Autodesk Inventor part; units mm, degrees
ref_plane "YZ Plane" through (0, 0, 0) normal (1, 0, 0) x (0, 1, 0)
ref_plane "XZ Plane" through (0, 0, 0) normal (0, 1, 0) x (-1, 0, 0)
ref_plane "XY Plane" through (0, 0, 0) normal (0, 0, 1) x (1, 0, 0)
sketch "Sketch1" plane through (0, 0, 0) normal (1, 0, 0) x (0, 1, 0)
  line L0 (6.2348, 11.9337) -> (6.2348, 11.9337)
  line L1 (2.2348, 7.9337) -> (2.2348, -14.0663)
  line L2 (6.2348, -18.0663) -> (6.2348, -18.0663)
  line L3 (10.2348, -14.0663) -> (10.2348, 7.9337)
  circle A0 centre (6.2348, 6.9337) radius 1.25
  circle A1 centre (6.2348, -3.0663) radius 1.25
  circle A2 centre (6.2348, -13.0663) radius 2.25
  arc A3 (6.2348, -18.0663) -> (10.2348, -14.0663) centre (6.2348, -14.0663) ccw
  arc A4 (2.2348, -14.0663) -> (6.2348, -18.0663) centre (6.2348, -14.0663) ccw
  arc A5 (6.2348, 11.9337) -> (2.2348, 7.9337) centre (6.2348, 7.9337) ccw
  arc A6 (10.2348, 7.9337) -> (6.2348, 11.9337) centre (6.2348, 7.9337) ccw
  point P0 (0, 0)
  point P1 (10.2348, 11.9337)
  point P2 (2.2348, 11.9337)
  point P3 (10.2348, -18.0663)
  dimension "d0" = 30
  dimension "d1" = 8
  dimension "d2" = 10
  dimension "d3" = 20
  dimension "d4" = 5
  dimension "d5" = 4.5
  dimension "d6" = 2.5
  dimension "d7" = 2.5
  dimension "d8" = 4
extrude "Extrusion1" add sketch "Sketch1" along normal blind 2
sketch "Sketch2" plane through (2, 0, 0) normal (1, 0, 0) x (0, 0, -1)
  circle A0 centre (-1.9337, 6.2348) radius 2
  circle A1 centre (3.0663, 6.2348) radius 1.25
  point P0 (0, 0)
  dimension "d11" = 4
  dimension "d12" = 5
extrude "Extrusion2" add sketch "Sketch2" along normal blind 10 contours A0
fillet "Fillet1" radius 1 1 edges at (2, 6.2348, 3.9337)
sketch "Sketch4" plane through (2, 0, 0) normal (1, 0, 0) x (0, 0, -1)
  circle A0 centre (13.0663, 6.2348) radius 2.25
  circle A1 centre (13.0663, 6.2348) radius 2.4
  point P0 (0, 0)
  dimension "d25" = 4.8
extrude "Extrusion4" add sketch "Sketch4" along normal blind 9 and the other way blind 2 contours A0
fillet "Fillet2" radius 1 1 edges at (11, 6.2348, -10.8163)
properties part number "cube_Holder"
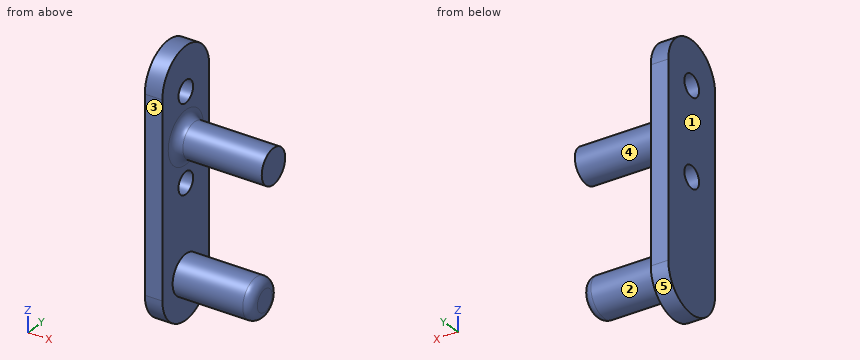
Geometry check sheet. Reference: the model listing, model coordinates, mm. Face numbers are marked on the shaded views. A direction names the side the tool comes from. Round coordinates to 2 decimals unless told otherwise and drop trailing zeros. Loops run counter-clockwise (first coordinate to the right, second up) from the corner with the lowest first, then second, coordinate; pieces in that order, holes last. Notation, with made-up numbers: M -20.5,-10 L 30.5,-10 A30 cw 30.5,13 Z; hole C 7,-29 d1. An arc over 180 degrees is marked long. Return JSON: item names as keys, results as strings. Group by question number.
(1) Section check C-C, the plane y = 5.5. Give the number of separate pieces and of enclosed holes in the cut face, and give its area (3 significant figures).
(2) Mould release check, pull along Z, two halves, no side actions. Record for the marked faces 3, 4 and 5: pulls with the +Z half, pulls with the -Z half, needs draft (parallel to the pull), parting line crosses it, or undercut.
(3) Section check B-B, the plane x = 4. Enter the section's corners in (y, z), and give its area (3 significant figures).
(4) Section check D-D, the plane z = -6.5. Enter the section's corners in (x, y), and give its area (3 significant figures).
(5) Scan lines: line 1 along X through (y, z) = (6, -5); line 2 along Z through (x, y) = (2.25, 8.25); line 3 along Z through (x, y) = (3, 5.75). Record each from-to range of solid material in increasing order. Write a range as [from, to].
(6) Go/stop test with flat-tipped pins: pin 1 (1.5 mm diameter, centred on x = 10, y = 7, fed in from +Z); pin 2 (1 mm diameter, centred on x = 5, z = -14, fed in from -Y); pin 3 (3 mm diameter, centred on y = 6.23, z = -3.07, fed in from +X). Record where each tip stops, or that it passes through.
(7) Section check A-A, the plane z = 7.5. Enter the section's corners in (x, y).
(8) Set-up check for the marked faces 1 and 2: record each of +Z, -Z, +X, -X, +Y, -Y from which the full face is reachable in a straight line by a thin tool's end or side.
Data:
{
 "1": {"separate pieces": "3", "enclosed holes": "0", "area": "127 mm²"},
 "2": {"face 3": "needs draft", "face 4": "undercut", "face 5": "pulls with the -Z half"},
 "3": {"outline": "C 6.23,-13.07 d4.5; C 6.23,1.93 d4", "area": "28.5 mm²"},
 "4": {"outline": "M 0,2.23 L 2,2.23 L 2,10.23 L 0,10.23 Z", "area": "16.0 mm²"},
 "5": {"line 1": "[0, 2]", "line 2": "[-14.07, -12.07], [0.75, 3.12]", "line 3": "[-15.26, -10.87], [-0.01, 3.87]"},
 "6": {"pin 1": "z = 3.93", "pin 2": "y = 4.03", "pin 3": "x = 2"},
 "7": {"outline": "M 0,2.23 L 2,2.23 L 2,5.12 L 0,5.12 Z; M 0,7.35 L 2,7.35 L 2,10.23 L 0,10.23 Z"},
 "8": {"face 1": "+Z, -Z, -X, +Y, -Y", "face 2": "+X"}
}
